Input: part model. Units: mm. Frame: model coordinates. A direction names the side the tool comes from. Give positions to 0.01 mm unless a question says otherwise; leave off trailing zeros. Loops run counter-clockwise (first coordinate to the right, second up) from the corner with the lowest first, then second, coordinate; pieces in that order, holes last. Notation, with made-up numbers: M 73,83.25 L 120,83.25 A15 cw 120,97.25 Z; hole C 23,34.5 d3. An arc over 180 degrees is marked long. Use CSV: the item, a comma, the result in double quotes. Start each with the question number.
Q1. Section A-A, the plane y = 14.5. Output: boundary loops of the cut face in (x, z).
Q2. Section C-C, the plane z = 2. Output: boundary loops of the cut face in (x, y).
Q3. Pull-direction query (X, two-part tool) for faces 1 (the flat face through (-174, -14, 4)), 2 (the flat face through (-111.5, -21, 4)), 3 (the flat face through (-2, -66, 8)); classes: released by +X, released by -X, zero draft, split by the parting line, or undercut.
Q4. Section D-D, the plane x = 41. Output: boundary loops of the cut face in (y, z), plus the area to 3 significant figures.
Q5. Material intervals for line 1 along X through (y, z) = (-30, 6); line 2 along X through (y, z) = (-14.5, 6); line 3 along X through (y, z) = (-9, 6), sorted ascending.
Q6. Section B-B, the plane y = -25. Output: boundary loops of the cut face in (x, z), plus the area to 3 significant figures.
Q7. Pin query (flat end, axial travel): pin 1 (2 mm diameter, centred on y = -60.5, z = 1, fed in from +X); pin 2 (4 mm diameter, centred on x = -171, z = 2.5, fed in from +Y); pin 3 (4 mm diameter, centred on y = -63.5, z = 2.5, fed in from -X). Return the tip coordinate at first contact, or that it passes through.
Q8. Reachability of faces 4 (the flat face through (170, -34.5, 4)), 5 (the flat face through (170, 5.5, 4)), 6 (the cylindrical face through (-126.72, 25.12, 4.06)), 7 (the flat face through (-170, -34.5, 4)) from +Z, -Z, +X, -X, +Y, -Y: full face, straight path, thin tool, end or side. Return the list, or none.
Autodesk Inventor part; units mm, degrees
ref_plane "YZ Plane" through (0, 0, 0) normal (1, 0, 0) x (0, 1, 0)
ref_plane "XZ Plane" through (0, 0, 0) normal (0, 1, 0) x (-1, 0, 0)
ref_plane "XY Plane" through (0, 0, 0) normal (0, 0, 1) x (1, 0, 0)
sketch "Эскиз1" plane through (0, 0, 0) normal (0, 0, 1) x (1, 0, 0)
  line L0 (-166, 74.5) -> (166, 74.5)
  line L1 (166, 74.5) -> (166, -74.5)
  line L2 (166, -74.5) -> (-166, -74.5)
  line L3 (-166, -74.5) -> (-166, 74.5)
  point P0 (0, 0)
  dimension "d0" = 332
  dimension "d1" = 149
  dimension "d3" = 166
  dimension "d4" = 74.5
extrude "Выдавливание1" add sketch "Эскиз1" along normal blind 8
sketch "Эскиз2" plane through (0, 0, 8) normal (0, 0, 1) x (1, 0, 0)
  line L0 (166, 74.5) -> (-166, 74.5)
  line L1 (-166, -74.5) -> (166, -74.5)
  circle A0 centre (0, 74.5) radius 136
  point P0 (0, 0)
  point P1 (-136, 74.5)
  point P2 (136, 74.5)
  dimension "d8" = 272
extrude "Выдавливание2" cut sketch "Эскиз2" against normal through all contours A0 L0 picked at (19.0214, 16.0372)
sketch "Эскиз3" plane through (0, 0, 8) normal (0, 0, 1) x (1, 0, 0)
  line L0 (103.5, -3.3701) -> (111.5, -3.3701)
  line L1 (111.5, -3.3701) -> (111.5, -38)
  line L2 (111.5, -38) -> (103.5, -38)
  line L3 (103.5, -38) -> (103.5, -3.3701)
  line L4 (-111.5, -3.3701) -> (-103.5, -3.3701)
  line L5 (-103.5, -3.3701) -> (-103.5, -38)
  line L6 (-103.5, -38) -> (-111.5, -38)
  line L7 (-111.5, -38) -> (-111.5, -3.3701)
  line L8 (166, -74.5) -> (166, 74.5)
  line L9 (-166, -74.5) -> (166, -74.5)
  line L10 (-166, 74.5) -> (-166, -74.5)
  arc A0 (-136, 74.5) -> (136, 74.5) centre (0, 74.5) ccw
  point P0 (0, 0)
  dimension "d11" = 54.5
  dimension "d12" = 36.5
  dimension "d13" = 54.5
  dimension "d14" = 36.5
  dimension "d15" = 8
  dimension "d16" = 8
extrude "Выдавливание3" cut sketch "Эскиз3" against normal through all
sketch "Эскиз4" plane through (-166, -74.5, 0) normal (-1, 0, 0) x (0, 0, 1)
  line L0 (0, 80) -> (8, 80)
  line L1 (8, 80) -> (8, 40)
  line L2 (8, 40) -> (0, 40)
  line L3 (0, 40) -> (0, 80)
  line L4 (0, 0) -> (8, 0)
  line L5 (0, 149) -> (0, 0)
  point P0 (0, 74.5)
  dimension "d19" = 40
  dimension "d20" = 40
  dimension "d21" = 8
  dimension "d22" = 0
extrude "Выдавливание4" add sketch "Эскиз4" along normal blind 8
sketch "Эскиз5" plane through (166, -74.5, 0) normal (1, 0, 0) x (0, 0, -1)
  line L0 (-8, 80) -> (0, 80)
  line L1 (0, 80) -> (0, 40)
  line L2 (0, 40) -> (-8, 40)
  line L3 (-8, 40) -> (-8, 80)
  line L4 (0, 0) -> (-8, 0)
  line L5 (-8, 0) -> (-8, 149)
  point P0 (0, 74.5)
  dimension "d25" = 40
  dimension "d26" = 40
  dimension "d27" = 0
  dimension "d28" = 8
extrude "Выдавливание5" add sketch "Эскиз5" along normal blind 8
sketch "Эскиз6" plane through (0, 0, 8) normal (0, 0, 1) x (1, 0, 0)
  line L0 (-136, 74.5) -> (-166, 74.5)
  line L1 (-166, 74.5) -> (-134.6663, 74.5)
  line L2 (-134.6663, 74.5) -> (-134.6663, 55.5)
  line L3 (-134.6663, 55.5) -> (-166, 55.5)
  line L4 (-166, 55.5) -> (-166, 74.5)
  line L5 (-166, 5.5) -> (-174, 5.5)
  arc A0 (-136, 74.5) -> (-111.5, -3.3701) centre (0, 74.5) ccw
  line L6 (166, 74.5) -> (136, 74.5)
  arc A1 (111.5, -3.3701) -> (136, 74.5) centre (0, 74.5) ccw
  line L7 (166, 74.5) -> (134.6663, 74.5)
  line L8 (134.6663, 74.5) -> (134.6663, 55.5)
  line L9 (134.6663, 55.5) -> (166, 55.5)
  line L10 (166, 55.5) -> (166, 74.5)
  line L11 (166, 5.5) -> (174, 5.5)
  point P0 (0, 0)
  dimension "d31" = 50
  dimension "d34" = 50
extrude "Выдавливание6" cut sketch "Эскиз6" against normal through all contours A0 L3 L4 L0 | L10 L9 A1 L6
sketch "Эскиз7" plane through (0, 0, 8) normal (0, 0, 1) x (1, 0, 0)
  line L0 (-166, 55.5) -> (-166, 5.5)
  line L1 (-166, 55.5) -> (-134.6663, 55.5)
  line L2 (-166, 5.5) -> (-139.6663, 55.5)
  line L3 (-139.6663, 55.5) -> (-160.2816, 66.3576)
  line L4 (-160.2816, 66.3576) -> (-186.6153, 16.3576)
  line L5 (-186.6153, 16.3576) -> (-166, 5.5)
  line L6 (166, 5.5) -> (166, 55.5)
  line L7 (166, 5.5) -> (139.6663, 55.5)
  line L8 (139.6663, 55.5) -> (160.2816, 66.3576)
  line L9 (160.2816, 66.3576) -> (186.6153, 16.3576)
  line L10 (186.6153, 16.3576) -> (166, 5.5)
  line L11 (166, 55.5) -> (134.6663, 55.5)
  line L12 (139.6663, 55.5) -> (134.6663, 55.5)
  arc A0 (-134.6663, 55.5) -> (-111.5, -3.3701) centre (0, 74.5) ccw
  line L13 (-139.6663, 55.5) -> (-134.6663, 55.5)
  point P0 (0, 0)
  dimension "d35" = 5
  dimension "d36" = 5
extrude "Выдавливание7" cut sketch "Эскиз7" against normal through all contours L1 L2 L0 | L7 L11 L6
properties part number "myDno"
A:
1,outline,"M -161.26,0 L -122.05,0 L -122.05,8 L -161.26,8 Z; M 122.05,0 L 161.26,0 L 161.26,8 L 122.05,8 Z"
2,outline,"M -174,-34.5 L -166,-34.5 L -166,-74.5 L 166,-74.5 L 166,-34.5 L 174,-34.5 L 174,5.5 L 166,5.5 L 139.67,55.5 L 134.67,55.5 A136 cw 111.5,-3.37 L 111.5,-38 L 103.5,-38 L 103.5,-13.73 A136 cw -103.5,-13.73 L -103.5,-38 L -111.5,-38 L -111.5,-3.37 A136 cw -134.67,55.5 L -139.67,55.5 L -166,5.5 L -174,5.5 Z"
3,face 1,"released by -X"
3,face 2,"undercut"
3,face 3,"zero draft"
4,outline,"M -74.5,0 L -55.17,0 L -55.17,8 L -74.5,8 Z"
4,area,"155 mm^2"
5,line 1,"-174 to -111.5, -103.5 to -87.04, 87.04 to 103.5, 111.5 to 174"
5,line 2,"-174 to -111.5, -103.5 to -102.83, 102.83 to 103.5, 111.5 to 174"
5,line 3,"-174 to -111.5, 111.5 to 174"
6,outline,"M -174,0 L -111.5,0 L -111.5,8 L -174,8 Z; M -103.5,0 L -92.71,0 L -92.71,8 L -103.5,8 Z; M 92.71,0 L 103.5,0 L 103.5,8 L 92.71,8 Z; M 111.5,0 L 174,0 L 174,8 L 111.5,8 Z"
6,area,"1,170 mm^2"
7,pin 1,"x = 166"
7,pin 2,"y = 5.5"
7,pin 3,"x = -166"
8,face 4,"+Z, -Z, +X, -Y"
8,face 5,"+Z, -Z, +X, +Y"
8,face 6,"+Z, -Z, +Y"
8,face 7,"+Z, -Z, -X, -Y"
